from build123d import *

# Parameters (mm, degrees)
SKETCH1_R           = 2.9
SKETCH1_R_2         = 2
BOSS_EXTRUDE1_DEPTH = 5


with BuildPart() as part:
    # Sketch1 → Boss-Extrude1 (new body)
    with BuildSketch(Plane(origin=(0, 0, 0), x_dir=(1, 0, 0), z_dir=(0, 1, 0))):
        with BuildLine():
            Line((-5, 40), (-7.87901938, 0.575372577))
            ThreePointArc((-7.87901938, 0.575372577), (-0.287877487, -7.894753103), (7.9, 0))
            Line((7.9, 0), (7.817385493, 1.139510448))
            Line((7.817385493, 1.139510448), (5, 40))
            ThreePointArc((5, 40), (0, 45), (-5, 40))
        make_face()
        with Locations(Location((0, 0, 0), (0, 0, 270))):
            Circle(SKETCH1_R, mode=Mode.SUBTRACT)
        with Locations(Location((0, 40, 0), (0, 0, 270))):
            Circle(SKETCH1_R_2, mode=Mode.SUBTRACT)
    extrude(amount=BOSS_EXTRUDE1_DEPTH)


solid = part.part
Can you work these out from the model? Positions are in its coordinate system, mm. Give positions to 0.01 mm unless a question says otherwise; leave off trailing zeros. Loops run counter-clockwise (first coordinate to the right, second up) from the corner with the lowest first, then second, coordinate; pieces in that order, holes last. Notation, with made-up numbers: M 66.25,28.5 L 124.25,28.5 A19 cw 124.25,60.5 Z; hole C -30,62 d4. An arc over 180 degrees is marked long. One line per item, written item: value.
1) Imagine slicing it at B-B on y = 1.45. Write out the boundary of the cut face in (x, z), and give its area (3 significant figures).
Geometry check:
outline: M -7.88,-0.58 L -5,-40 A5 ccw 5,-40 L 7.9,0 A7.9 ccw long Z; hole C 0,0 d5.8; hole C 0,-40 d4
area: 615 mm²
2) Thinking about a two-plate mould opening in Z: for faces 1 (the face through (0, 5, -19)), 2 (the face through (0, 2, -42)), 3 (the face through (0, 2, -45)), 4 (the face through (0.1, 2.5, -2.9)), which applies, +Z half, -Z half, draft (parallel to the pull), parting line (faces both ways), or undercut?
Geometry check:
face 1: draft
face 2: undercut
face 3: -Z half
face 4: undercut
3) Imagine slicing it at C-C on z = -24.5. Write out the boundary of the cut face in (x, y).
Geometry check:
outline: M -6.13,0 L 6.12,0 L 6.12,5 L -6.13,5 Z
4) Please list where these lines run through material, in increasing order: line 1 (X direction, y = 3.3, z = -40); line 2 (Z direction, x = -1.25, y = 0.9); line 3 (Z direction, x = 0.75, y = 0.3).
Geometry check:
line 1: x = -5 to -2, 2 to 5
line 2: z = -44.84 to -41.56, -38.44 to -2.62, 2.62 to 7.8
line 3: z = -44.94 to -41.85, -38.15 to -2.8, 2.8 to 7.86
5) I'm going to push flat-ended pins straight in: pin 1 (1.5 mm diameter, centred on y = 4, z = -31.5, fed in from +X); pin 2 (1.5 mm diameter, centred on y = 4, z = -28, fed in from +X); pin 3 (1.5 mm diameter, centred on x = 0, z = -22.5, fed in from -Y); pin 4 (1 mm diameter, centred on y = 3.5, z = -35.5, fed in from -X). Where does each tip first touch, or does it pass through?
Geometry check:
pin 1: stops at x = 5.67
pin 2: stops at x = 5.92
pin 3: stops at y = 0
pin 4: stops at x = -5.37
6) Imagine slicing it at A-A on x = 0. Write out the boundary of the cut face in (y, z), and give its area (4 significant figures).
Geometry check:
outline: M 0,-45 L 5,-45 L 5,-42 L 0,-42 Z; M 0,-38 L 5,-38 L 5,-2.9 L 0,-2.9 Z; M 0,2.9 L 5,2.9 L 5,7.9 L 0,7.9 Z
area: 215.5 mm²
7) Imagine slicing it at D-D on x = 3.75. Write out the boundary of the cut face in (y, z).
Geometry check:
outline: M 0,-43.31 L 5,-43.31 L 5,6.95 L 0,6.95 Z
